Could you check a few things on this model? Use its own coordinates, in mm. A direction names the side the tool comes from. Round coordinates to 2 decimals unless told otherwise and drop trailing zeros. Write each loop counter-clockwise with the first axis right and the second up, starting at its lowest first coordinate (ties: lowest second). Pieces come first, ordered by that corner, then holes. Notation, with made-up numbers: M -38.75,14 L -25.75,14 A34 cw -25.75,51 Z; hole C 86.5,57 d9. An arc over 180 degrees is marked long. One line per item, written item: value. Start each with the question number.
(1) Thinking about a two-plate mould opening in X: for faces 1 (the face through (-1.301, -45.857, 7.746)), 2 (the face through (-12.5, 50, -3)), 3 (the face through (12.5, -45, -12)), which applies, released by +X, released by -X, zero draft, split by the parting line, or undercut?
(2) If I drill on L1, parallel to Y at x = 0, z = -2; L2, parallel to Y at x = 0, z = -11.15; L3, parallel to X at y = 50, z = -13, over which ranges is the centre line in solid material (lowest first)?
(3) I want a section at C-C on y = -69. Please give me the cut outline in (x, z), and give its area (3 significant figures).
(4) I want a section at D-D on y = -40. Please give me the cut outline in (x, z), and give its area (3 significant figures).
(5) I want a section at A-A on z = -15.5. Please give me the cut outline in (x, y), and give its area (3 significant figures).
(6) Which directions (+Z, -Z, +X, -X, +Y, -Y) give clear straight access to the entire face, cutting with the end or side of a thin tool? Please do faces 4 (the face through (0, 29, -3)), 5 (the face through (-0.739, -40, 6)), 6 (the face through (0, 42, -20)), 7 (the face through (0, 75, -3)), 8 (the face through (15.59, 78.06, 6.48)).
(7) I want a section at B-B on y = 31. Please give me the cut outline in (x, z).
(8) I'm going to push flat-ended pins straight in: pin 1 Ø4 at (x, y) = (-9, -16.5) entering from -Z; pin 2 Ø1.5 at (y, z) = (40.5, -7.5) entering from +X; pin 3 Ø3 at (x, y) = (0.5, 31.5) entering from +Z. Where does each tip first touch, or does it pass through?
```python
from build123d import *

# Parameters (mm, degrees)
SKETCH_1_W            = 35
SKETCH_1_H            = 160
EXTRUDE_1_DEPTH       = 8
FILLET_1_R            = 3
CHAMFER_1_SIZE        = 3
CUT_EXTRUDE_1_DEPTH   = 0.5
SKETCH_3_R            = 6
EXTRUDE_2_DEPTH       = 0.5
SKETCH_4_W            = 25
SKETCH_4_H            = 150
EXTRUDE_3_DEPTH       = 24
SKETCH_6_W            = 25
SKETCH_6_H            = 50
CUT_EXTRUDE_3_DEPTH   = 24
SKETCH_8_W            = 10
SKETCH_8_H            = 15
CUT_EXTRUDE_4_DEPTH   = 89.746830929
SKETCH_9_W            = 25
SKETCH_9_H            = 50
SKETCH_9_R            = 10.35
CUT_EXTRUDE_5_DEPTH   = 24
SKETCH_10_R           = 2
CUT_EXTRUDE_6_DEPTH   = 4
SKETCH_11_W           = 25
SKETCH_11_H           = 50
EXTRUDE_2_2_DEPTH     = 7
SKETCH_12_W           = 1.47707906
SKETCH_12_H           = 9.426983126
CUT_EXTRUDE_7_DEPTH   = 5
HOLE_WIZARD_M61_D     = 5
HOLE_WIZARD_M61_DEPTH = 17
HOLE_WIZARD_M61_TIP   = 1.502151548
SKETCH_16_R           = 2
CUT_EXTRUDE_8_DEPTH   = 7.5
SKETCH_17_R           = 10.35
SKETCH_17_W           = 8
SKETCH_17_H           = 8
CUT_EXTRUDE_9_DEPTH   = 2.5
CUT_EXTRUDE_10_DEPTH  = 3.5


with BuildPart() as part:
    # Эскиз1 → Вытянуть1 (new body)
    with BuildSketch(Plane.XY):
        Rectangle(SKETCH_1_W, SKETCH_1_H)
    extrude(amount=EXTRUDE_1_DEPTH)

    # Скругление1
    fillet_1_edges = [part.edges().sort_by_distance(p)[0] for p in [
        (-17.5, 80, 4),
        (17.5, 80, 4),
        (17.5, -80, 4),
        (-17.5, -80, 4),
    ]]
    fillet(fillet_1_edges, radius=FILLET_1_R)

    # Фаска1
    chamfer_1_edges = [part.edges().sort_by_distance(p)[0] for p in [
        (0, -80, 8),
        (-17.5, 0, 8),
        (17.5, 0, 8),
        (0, 80, 8),
        (16.621320344, 79.121320344, 8),
        (-16.621320344, 79.121320344, 8),
        (16.621320344, -79.121320344, 8),
        (-16.621320344, -79.121320344, 8),
    ]]
    chamfer(chamfer_1_edges, length=CHAMFER_1_SIZE)

    # Эскиз2 → Вырез-Вытянуть1 (cut)
    with BuildSketch(Plane.XY.offset(8)):
        with BuildLine():
            Line((-9, 50), (-9, -50))
            ThreePointArc((-9, -50), (0, -59), (9, -50))
            Line((9, -50), (9, 50))
            ThreePointArc((9, 50), (0, 59), (-9, 50))
        make_face()
    extrude(amount=-CUT_EXTRUDE_1_DEPTH, mode=Mode.SUBTRACT)

    # Эскиз3 → Extrude 2 (add)
    with BuildSketch(Plane.XY.offset(7.5)):
        with Locations((0, -40)):
            Circle(SKETCH_3_R)
    extrude(amount=EXTRUDE_2_DEPTH)

    # Эскиз4 → Вытянуть3 (add)
    with BuildSketch(Plane(origin=(0, 0, 0), x_dir=(-1, 0, 0), z_dir=(0, 0, -1))):
        Rectangle(SKETCH_4_W, SKETCH_4_H)
    extrude(amount=EXTRUDE_3_DEPTH)

    # Эскиз6 → Вырез-Вытянуть3 (cut)
    with BuildSketch(Plane(origin=(0, 0, -24), x_dir=(-1, 0, 0), z_dir=(0, 0, -1))):
        Rectangle(SKETCH_6_W, SKETCH_6_H)
    extrude(amount=-CUT_EXTRUDE_3_DEPTH, mode=Mode.SUBTRACT)

    # Эскиз8 → Вырез-Вытянуть4 (cut, through all)
    with BuildSketch(Plane(origin=(12.5, 0, 0), x_dir=(0, 0, -1), z_dir=(1, 0, 0))):
        with Locations((19, -67.5)):
            Rectangle(SKETCH_8_W, SKETCH_8_H)
    extrude(amount=-CUT_EXTRUDE_4_DEPTH, mode=Mode.SUBTRACT)

    # Эскиз9 → Вырез-Вытянуть5 (cut)
    with BuildSketch(Plane(origin=(0, 0, -24), x_dir=(-1, 0, 0), z_dir=(0, 0, -1))):
        with Locations((0, 50)):
            Rectangle(SKETCH_9_W, SKETCH_9_H)
        with Locations((0, 50)):
            Circle(SKETCH_9_R, mode=Mode.SUBTRACT)
    extrude(amount=-CUT_EXTRUDE_5_DEPTH, mode=Mode.SUBTRACT)

    # Эскиз10 → Вырез-Вытянуть6 (cut)
    with BuildSketch(Plane(origin=(0, 0, -14), x_dir=(-1, 0, 0), z_dir=(0, 0, -1))):
        with Locations((0, -69)):
            Circle(SKETCH_10_R)
    extrude(amount=-CUT_EXTRUDE_6_DEPTH, mode=Mode.SUBTRACT)

    # Эскиз11 → Extrude 2 2 (add)
    with BuildSketch(Plane(origin=(0, 0, 0), x_dir=(-1, 0, 0), z_dir=(0, 0, -1))):
        with Locations((0, 50)):
            Rectangle(SKETCH_11_W, SKETCH_11_H)
    extrude(amount=EXTRUDE_2_2_DEPTH)

    # Эскиз12 → Вырез-Вытянуть7 (cut)
    with BuildSketch(Plane.XY.offset(8)):
        with Locations((0, -40)):
            Rectangle(SKETCH_12_W, SKETCH_12_H)
        with BuildLine():
            ThreePointArc((0.73853953, -42.00191483), (1.817071347, -39.86854196), (0.73853953, -37.73516909))
            Line((0.73853953, -37.73516909), (0.73853953, -42.00191483))
        make_face()
    extrude(amount=-CUT_EXTRUDE_7_DEPTH, mode=Mode.SUBTRACT)

    # Отверстие обработанное метчиком M61
    with Locations(Plane(origin=(0, 0, -24), x_dir=(-1, 0, 0), z_dir=(0, 0, -1))):
        with Locations((0, 50)):
            Hole(HOLE_WIZARD_M61_D / 2, depth=HOLE_WIZARD_M61_DEPTH)
            with Locations((0, 0, -(HOLE_WIZARD_M61_DEPTH + HOLE_WIZARD_M61_TIP / 2))):  # 118° drill point
                Cone(0, HOLE_WIZARD_M61_D / 2, HOLE_WIZARD_M61_TIP, mode=Mode.SUBTRACT)

    # Эскиз16 → Вырез-Вытянуть8 (cut)
    with BuildSketch(Plane(origin=(0, 0, -7), x_dir=(-1, 0, 0), z_dir=(0, 0, -1))):
        with Locations((0, 31)):
            Circle(SKETCH_16_R)
        with Locations(Location((0, 69, 0), (0, 0, 180))):
            Circle(SKETCH_16_R)
    extrude(amount=-CUT_EXTRUDE_8_DEPTH, mode=Mode.SUBTRACT)

    # Эскиз17 → Вырез-Вытянуть9 (cut)
    with BuildSketch(Plane(origin=(0, 0, -24), x_dir=(-1, 0, 0), z_dir=(0, 0, -1))):
        with Locations((0, 50)):
            Circle(SKETCH_17_R)
        with Locations((0, 50)):
            Rectangle(SKETCH_17_W, SKETCH_17_H, mode=Mode.SUBTRACT)
    extrude(amount=-CUT_EXTRUDE_9_DEPTH, mode=Mode.SUBTRACT)

    # Эскиз18 → Вырез-Вытянуть10 (cut)
    with BuildSketch(Plane(origin=(0, 0, -21.5), x_dir=(-1, 0, 0), z_dir=(0, 0, -1))):
        with BuildLine():
            Line((0, 44.343145751), (0, 39.65))
            ThreePointArc((0, 39.65), (7.318555185, 42.681444815), (10.35, 50))
            Line((10.35, 50), (5.656854249, 50))
            ThreePointArc((5.656854249, 50), (4, 46), (0, 44.343145751))
        make_face()
    extrude(amount=-CUT_EXTRUDE_10_DEPTH, mode=Mode.SUBTRACT)


solid = part.part
```
Found:
1. face 1: undercut
1. face 2: released by -X
1. face 3: released by +X
2. L1: y = -75 to -25, 25 to 29, 33 to 67, 71 to 75
2. L2: y = -75 to -71, -67 to -25, 39.65 to 47.5, 52.5 to 60.35
2. L3: x = -10.35 to -2.5, 2.5 to 10.35
3. outline: M -17.5,0 L -12.5,0 L -12.5,-14 L -2,-14 L -2,-10 L 2,-10 L 2,-14 L 12.5,-14 L 12.5,0 L 17.5,0 L 17.5,5 L 14.5,8 L -14.5,8 L -17.5,5 Z
3. area: 605 mm²
4. outline: M -17.5,0 L -12.5,0 L -12.5,-24 L 12.5,-24 L 12.5,0 L 17.5,0 L 17.5,5 L 14.5,8 L 9,8 L 9,7.5 L 6,7.5 L 6,8 L 1.81,8 L 1.81,3 L -0.74,3 L -0.74,8 L -6,8 L -6,7.5 L -9,7.5 L -9,8 L -14.5,8 L -17.5,5 Z
4. area: 855 mm²
5. outline: M -12.5,-60 L 12.5,-60 L 12.5,-25 L -12.5,-25 Z; C 0,50 d20.7; hole C 0,50 d5
5. area: 1,190 mm²
6. face 4: -Z
6. face 5: +Z
6. face 6: -Z, -X
6. face 7: -Z, +X, -X, +Y
6. face 8: +Z, +X, +Y
7. outline: M -17.5,0 L -12.5,0 L -12.5,-7 L -2,-7 L -2,0.5 L 2,0.5 L 2,-7 L 12.5,-7 L 12.5,0 L 17.5,0 L 17.5,5 L 14.5,8 L 9,8 L 9,7.5 L -9,7.5 L -9,8 L -14.5,8 L -17.5,5 Z
8. pin 1: stops at z = 0
8. pin 2: stops at x = 12.5
8. pin 3: stops at z = 7.5
